from build123d import *

# Parameters (mm, degrees)
SKETCH1_W                    = 40
SKETCH1_H                    = 800
BASE_FLANGE1_DEPTH           = 2
EDGE_FLANGE1_STRIP_W         = 9.4732
EDGE_FLANGE1_STRIP_H         = 2
EDGE_FLANGE1_STRIP_CUT_DEPTH = 800
EDGE_FLANGE1_DEPTH           = 800
EDGE_FLANGE2_STRIP_W         = 9.4732
EDGE_FLANGE2_STRIP_H         = 2
EDGE_FLANGE2_STRIP_CUT_DEPTH = 800
EDGE_FLANGE2_DEPTH           = 800
EDGE_FLANGE3_STRIP_W         = 9.4732
EDGE_FLANGE3_STRIP_H         = 2
EDGE_FLANGE3_STRIP_CUT_DEPTH = 800
EDGE_FLANGE3_DEPTH           = 800
EDGE_FLANGE4_STRIP_W         = 9.4732
EDGE_FLANGE4_STRIP_H         = 2
EDGE_FLANGE4_STRIP_CUT_DEPTH = 800
EDGE_FLANGE4_DEPTH           = 800
SKETCH20_R                   = 3
CUT_EXTRUDE1_DEPTH           = 414.067791046


# Sheet-metal steps are written as plain solids
with BuildPart() as part:
    # Sketch1 → Base-Flange1 (new body)
    with BuildSketch(Plane.XY):
        Rectangle(SKETCH1_W, SKETCH1_H)
    extrude(amount=-BASE_FLANGE1_DEPTH)

    # Edge-Flange1 strip (across the edge) → Edge-Flange1 strip cut (cut)
    with BuildSketch(Plane(origin=(20, 400, -2), x_dir=(-1, 0, 0), z_dir=(0, -1, 0))):
        with Locations((-2, -1)):
            Rectangle(EDGE_FLANGE1_STRIP_W, EDGE_FLANGE1_STRIP_H)
    extrude(amount=EDGE_FLANGE1_STRIP_CUT_DEPTH, mode=Mode.SUBTRACT)

    # Edge-Flange1 section (across the edge) → Edge-Flange1 (add)
    with BuildSketch(Plane(origin=(20, 400, -2), x_dir=(-1, 0, 0), z_dir=(0, -1, 0))):
        with BuildLine():
            Line((0, 0.7366), (0, 11))
            Line((0, 11), (2, 11))
            Line((2, 11), (2, 0.7366))
            ThreePointArc((2, 0.7366), (2.215745145, 0.215745145), (2.7366, 0))
            Line((2.7366, 0), (2.7366, -2))
            ThreePointArc((2.7366, -2), (0.801531583, -1.198468417), (0, 0.7366))
        make_face()
    extrude(amount=EDGE_FLANGE1_DEPTH)

    # Edge-Flange2 strip (across the edge) → Edge-Flange2 strip cut (cut)
    with BuildSketch(Plane(origin=(18, 400, -13), x_dir=(0, 0, 1), z_dir=(0, -1, 0))):
        with Locations((-2, -1)):
            Rectangle(EDGE_FLANGE2_STRIP_W, EDGE_FLANGE2_STRIP_H)
    extrude(amount=EDGE_FLANGE2_STRIP_CUT_DEPTH, mode=Mode.SUBTRACT)

    # Edge-Flange2 section (across the edge) → Edge-Flange2 (add)
    with BuildSketch(Plane(origin=(18, 400, -13), x_dir=(0, 0, 1), z_dir=(0, -1, 0))):
        with BuildLine():
            Line((0, 0.7366), (0, 38))
            Line((0, 38), (2, 38))
            Line((2, 38), (2, 0.7366))
            ThreePointArc((2, 0.7366), (2.215745145, 0.215745145), (2.7366, 0))
            Line((2.7366, 0), (2.7366, -2))
            ThreePointArc((2.7366, -2), (0.801531583, -1.198468417), (0, 0.7366))
        make_face()
    extrude(amount=EDGE_FLANGE2_DEPTH)

    # Edge-Flange3 strip (across the edge) → Edge-Flange3 strip cut (cut)
    with BuildSketch(Plane(origin=(-20, -400, -13), x_dir=(1, 0, 0), z_dir=(0, 1, 0))):
        with Locations((-2, -1)):
            Rectangle(EDGE_FLANGE3_STRIP_W, EDGE_FLANGE3_STRIP_H)
    extrude(amount=EDGE_FLANGE3_STRIP_CUT_DEPTH, mode=Mode.SUBTRACT)

    # Edge-Flange3 section (across the edge) → Edge-Flange3 (add)
    with BuildSketch(Plane(origin=(-20, -400, -13), x_dir=(1, 0, 0), z_dir=(0, 1, 0))):
        with BuildLine():
            Line((0, 0.7366), (0, 12))
            Line((0, 12), (2, 12))
            Line((2, 12), (2, 0.7366))
            ThreePointArc((2, 0.7366), (2.215745145, 0.215745145), (2.7366, 0))
            Line((2.7366, 0), (2.7366, -2))
            ThreePointArc((2.7366, -2), (0.801531583, -1.198468417), (0, 0.7366))
        make_face()
    extrude(amount=EDGE_FLANGE3_DEPTH)

    # Edge-Flange4 strip (across the edge) → Edge-Flange4 strip cut (cut)
    with BuildSketch(Plane(origin=(-18, -400, -25), x_dir=(0, 0, 1), z_dir=(0, 1, 0))):
        with Locations((-2, -1)):
            Rectangle(EDGE_FLANGE4_STRIP_W, EDGE_FLANGE4_STRIP_H)
    extrude(amount=EDGE_FLANGE4_STRIP_CUT_DEPTH, mode=Mode.SUBTRACT)

    # Edge-Flange4 section (across the edge) → Edge-Flange4 (add)
    with BuildSketch(Plane(origin=(-18, -400, -25), x_dir=(0, 0, 1), z_dir=(0, 1, 0))):
        with BuildLine():
            Line((0, 0.7366), (0, 58))
            Line((0, 58), (2, 58))
            Line((2, 58), (2, 0.7366))
            ThreePointArc((2, 0.7366), (2.215745145, 0.215745145), (2.7366, 0))
            Line((2.7366, 0), (2.7366, -2))
            ThreePointArc((2.7366, -2), (0.801531583, -1.198468417), (0, 0.7366))
        make_face()
    extrude(amount=EDGE_FLANGE4_DEPTH)

    # Mirror2: part across plane


with BuildPart() as part_1:
    add(part.part)
    add(part.part.mirror(Plane(origin=(40, -400, -25), x_dir=(0, 0, 1), z_dir=(-1, 0, 0))))

    # Sketch20 → Cut-Extrude1 (cut, through all)
    with BuildSketch(Plane.XY):
        with Locations((90, 0)):
            Circle(SKETCH20_R)
        with Locations((90, 380)):
            Circle(SKETCH20_R)
        with Locations((90, -380)):
            Circle(SKETCH20_R)
        with Locations((-10, -380)):
            Circle(SKETCH20_R)
        with Locations((-10, 0)):
            Circle(SKETCH20_R)
        with Locations((-10, 380)):
            Circle(SKETCH20_R)
    extrude(amount=-CUT_EXTRUDE1_DEPTH, mode=Mode.SUBTRACT)


solid = part_1.part
Read the model definition and answer for the solid it produces. Units are mm, in the model's axes. A direction names the side the tool comes from. Round coordinates to 2 decimals unless told otherwise and drop trailing zeros. Order: outer loops, then holes, each group sorted by start corner. A loop starts at its lowest first (then second) coordinate and runs counter-clockwise, first axis right, second up.
1) The part is cut by section A-A on z = -17.75. Write down the section's boundary in (x, y).
2) For faces 5 (the face through (82, 6, -2)), 6 (the face through (0, 6, -11)), 7 (the face through (39, -6, -23)), determine the directions among +Z, -Z, +X, -X, +Y, -Y from which every point of the face is accessible in a straight line to the end or side of a thin tool.
3) The part is cut by section B-B on x = 52. Write down the section's boundary in (y, z), plus the area to 3 significant figures.
4) Straight lines are drawn through the part: L1, parallel to Y at x = 90, z = -12.2; L2, parallel to Z at x = 65, y = -109.5; L3, parallel to X at y = 311, z = -17.25. For each, find the intervals that lie inside material, in ascending order.
5) The mould has two halves that part along Z. Classify faces 1 (the face through (80, 6, -13)), 2 (the face through (40, -400, -24)), 3 (the face through (0, 6, -13)), 4 (the face through (82, 6, 0)): released by +Z, released by -Z, zero draft, split by the parting line, or undercut.
6) Flat-ended cylindrical pins translate along their axes: pin 1 (8 mm diameter, centred on x = 17, y = 89, fed in from +Z); pin 2 (6 mm diameter, centred on y = -116, z = -6.5, fed in from -X); pin 3 (4 mm diameter, centred on y = 203.5, z = -9.5, fed in from +X). Find the tip coordinate at first contact, or state that the pin passes through.
Resolved:
1. outline: (-20, -400) - (-18, -400) - (-18, 400) - (-20, 400) - close; (98, -400) - (100, -400) - (100, 400) - (98, 400) - close
2. face 5: +X, +Y, -Y
2. face 6: -X, +Y, -Y
2. face 7: +Y, -Y
3. outline: (-400, -25) - (400, -25) - (400, -23) - (-400, -23) - close
3. area: 1,600 mm2
4. L1: y = -400 to -383, -377 to -3, 3 to 377, 383 to 400
4. L2: z = -25 to -23, -13 to -11, -2 to 0
4. L3: x = -20 to -18, 98 to 100
5. face 1: undercut
5. face 2: zero draft
5. face 3: undercut
5. face 4: released by +Z
6. pin 1: stops at z = 0
6. pin 2: stops at x = 18
6. pin 3: stops at x = 98.84
